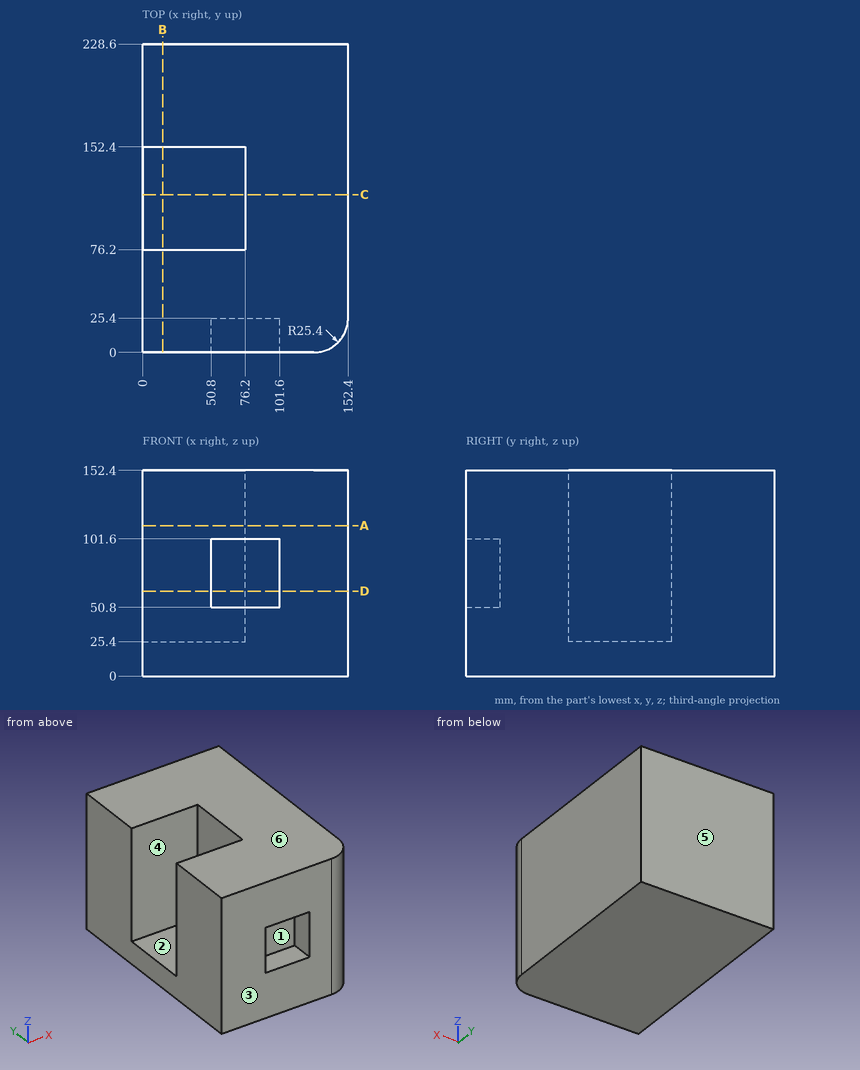
Source: three-view drawing plus pictorial views. Frame: mm from the lowest corner of the part. A direction names the side the tool comes from. Round coordinates to 2 decimals unless told otherwise and drop trailing zeros. Loops run counter-clockwise (first coordinate to the right, second up) from the corner with the lowest first, then second, coordinate; pieces in that order, holes last. Notation, with made-up numbers: M 64.25,27.5 L 87.25,27.5 A17 ccw 87.25,55.5 Z; hole C 46,-33.5 d8. An arc over 180 degrees is marked long. Put each result on its own line as item: value. Start each with the question number.
(1) Section query D-D (z = 63). Return loops of the section in (x, y), then the cut area to 3 significant figures.
(2) Material intervals for line 1 along Y through (x, z) = (10, 55.5); line 2 along Z through (x, y) = (56, 16); line 3 along X through (y, z) = (124.5, 128), sorted ascending. Write a range as [from, to].
(3) Set-up query: the marked faces 1, 2 and 3. Return all of +Z, -Z, +X, -X, +Y, -Y with unobstructed straight access to the full face (end or side cutting, diameter ignored); none if empty.
(4) Section query B-B (x = 15). Return loops of the section in (y, z), then the cut area to 3 significant figures.
(5) Section query A-A (z = 111.5). Return loops of the section in (x, y), then the cut area to 3 significant figures.
(6) Draft query along Y for the marked faces 4, 5 and 6. Return one class per face: +Y half, -Y half, draft (parallel to the pull), parting line (faces both ways), or undercut.
(7) Contact query for flat-ended pins moving along their axis: pin 1 Ø15 at (x, z) = (68, 84) entering from -Y; pin 2 Ø23 at (x, y) = (43, 115) entering from +Z. Output: stop coordinate, or through.
(8) Section query C-C (y = 117). Return loops of the section in (x, z).
Findings below:
1. outline: M 0,0 L 50.8,0 L 50.8,25.4 L 101.6,25.4 L 101.6,0 L 127,0 A25.4 ccw 152.4,25.4 L 152.4,228.6 L 0,228.6 L 0,152.4 L 76.2,152.4 L 76.2,76.2 L 0,76.2 Z
1. area: 27,600 mm2
2. line 1: y = [0, 76.2], [152.4, 228.6]
2. line 2: z = [0, 50.8], [101.6, 152.4]
2. line 3: x = [76.2, 152.4]
3. face 1: -Y
3. face 2: +Z, -X
3. face 3: +Z, -Z, +X, -X, -Y
4. outline: M 0,0 L 228.6,0 L 228.6,152.4 L 152.4,152.4 L 152.4,25.4 L 76.2,25.4 L 76.2,152.4 L 0,152.4 Z
4. area: 25,200 mm2
5. outline: M 0,0 L 127,0 A25.4 ccw 152.4,25.4 L 152.4,228.6 L 0,228.6 L 0,152.4 L 76.2,152.4 L 76.2,76.2 L 0,76.2 Z
5. area: 28,900 mm2
6. face 4: undercut
6. face 5: +Y half
6. face 6: draft
7. pin 1: stops at y = 25.4
7. pin 2: stops at z = 25.4
8. outline: M 0,0 L 152.4,0 L 152.4,152.4 L 76.2,152.4 L 76.2,25.4 L 0,25.4 Z
